from build123d import *

# Parameters (mm, degrees)
SKETCH1_W                = 12.14
SKETCH1_H                = 11.4
SKETCH1_R                = 0.9
BOSS_EXTRUDE1_DEPTH      = 1
BOSS_EXTRUDE2_DEPTH      = 1
BOSS_EXTRUDE2_DEPTH_BACK = 8
SKETCH1_3_W              = 24.28
SKETCH1_3_H              = 1


with BuildPart() as part:
    # Sketch1 → Boss-Extrude1 (new body)
    # profile 1 of 2: a face of its own
    with BuildSketch(Plane(origin=(0, 0, 0), x_dir=(1, 0, 0), z_dir=(0, 1, 0))):
        with Locations((6.07, 5.7)):
            Rectangle(SKETCH1_W, SKETCH1_H)
        with Locations(Location((1.5, 3, 0), (0, 0, 270))):
            Circle(SKETCH1_R, mode=Mode.SUBTRACT)
        with Locations(Location((1.5, 8, 0), (0, 0, 270))):
            Circle(SKETCH1_R, mode=Mode.SUBTRACT)
    # profile 2 of 2: a face of its own
    with BuildSketch(Plane(origin=(0, 0, 0), x_dir=(1, 0, 0), z_dir=(0, 1, 0))):
        with Locations((18.21, 5.7)):
            Rectangle(SKETCH1_W, SKETCH1_H)
        with Locations(Location((22.78, 3, 0), (0, 0, 270))):
            Circle(SKETCH1_R, mode=Mode.SUBTRACT)
        with Locations(Location((22.78, 8, 0), (0, 0, 270))):
            Circle(SKETCH1_R, mode=Mode.SUBTRACT)
    extrude(amount=BOSS_EXTRUDE1_DEPTH)

    # Sketch1_3 → Boss-Extrude2 (add, two sides: drawn at the far end of the back side and taken through both)
    with BuildSketch(Plane(origin=(0, 0, 0), x_dir=(1, 0, 0), z_dir=(0, 1, 0)).offset(-BOSS_EXTRUDE2_DEPTH_BACK)):
        with Locations((12.14, -0.5)):
            Rectangle(SKETCH1_3_W, SKETCH1_3_H)
    extrude(amount=BOSS_EXTRUDE2_DEPTH + BOSS_EXTRUDE2_DEPTH_BACK)


solid = part.part
Geometry: final body of the model. Coordinates: model frame, mm. A direction names the side the tool comes from. Round coordinates to 2 decimals unless told otherwise and drop trailing zeros. Order: outer loops, then holes, each group sorted by start corner. A loop starts at its lowest first (then second) coordinate and runs counter-clockwise, first axis right, second up. Notation, with made-up numbers: (62.5, -17.75) -> (79.5, -17.75) arc R17 ccw to (79.5, -13.75) -> close; hole circle Ø8 at (11, 46.5). An arc over 180 degrees is marked (long way). Put each result on its own line as item: value. Start each with the question number.
Q1. Section A-A on x = 22.78. Return the cut outline in (y, z), and give its area (3 significant figures).
Q2. Reachability of faces 1 (the flat face through (12, 1, -5)), 2 (the flat face through (12, -4, 0)) from +Z, -Z, +X, -X, +Y, -Y: full face, straight path, thin tool, end or side. Return the list, or none.
Q3. First-contact query: pin 1 (1.5 mm diameter, centred on x = 16, y = -6, fed in from -Z); pin 2 (1.6 mm diameter, centred on x = 22.78, z = -3, fed in from -Y); pin 3 (2.5 mm diameter, centred on x = 22.78, z = -8, fed in from -Y). Flat tips, straight axial feed; report the tip coordinate or a pass-through.
Q4. Section B-B on z = -3. Return the cut outline in (x, y), and give its area (3 significant figures).
Q5. Section D-D on y = -1.25. Return the cut outline in (x, z), and give its area (3 significant figures).
Q6. Pull-direction query (Z, two-part tool) for faces 3 (the flat face through (12, -4, 1)), 4 (the flat face through (24.28, 0.5, -2.9)), 5 (the cylindrical face through (21.901, 0.493, -3.195)); classes: +Z half, -Z half, draft (parallel to the pull), parting line (faces both ways), or undercut.
Q7. Line query: probe 1 along X at (y, z) = (0.25, -3); probe 2 along Z at (x, y) = (19.75, -0.25). Output: solid intervals per line, ascending.
Q8. Section C-C on x = 15. Return the cut outline in (y, z).
Ans:
1. outline: (-8, 0) -> (0, 0) -> (0, -2.1) -> (1, -2.1) -> (1, 1) -> (-8, 1) -> close; (0, -11.4) -> (1, -11.4) -> (1, -8.9) -> (0, -8.9) -> close; (0, -7.1) -> (1, -7.1) -> (1, -3.9) -> (0, -3.9) -> close
1. area: 16.8 mm2
2. face 1: +Z, -Z, +X, -X, +Y
2. face 2: -Z, +X, -X, -Y
3. pin 1: stops at z = 0
3. pin 2: passes through
3. pin 3: stops at y = 0
4. outline: (0, 0) -> (0.6, 0) -> (0.6, 1) -> (0, 1) -> close; (2.4, 0) -> (21.88, 0) -> (21.88, 1) -> (2.4, 1) -> close; (23.68, 0) -> (24.28, 0) -> (24.28, 1) -> (23.68, 1) -> close
4. area: 20.7 mm2
5. outline: (0, 0) -> (24.28, 0) -> (24.28, 1) -> (0, 1) -> close
5. area: 24.3 mm2
6. face 3: +Z half
6. face 4: draft
6. face 5: undercut
7. probe 1: x = 0 to 0.6, 2.4 to 21.88, 23.68 to 24.28
7. probe 2: z = 0 to 1
8. outline: (-8, 0) -> (0, 0) -> (0, -11.4) -> (1, -11.4) -> (1, 1) -> (-8, 1) -> close
